Can you work these out from the model? Positions are in its coordinate system, mm. A direction names the side the tool comes from. Coordinates: 2 decimals unless noted, no trailing zeros. Write each loop counter-clockwise with the first axis right and the second up, starting at its lowest first coordinate (ties: lowest second). Pieces come first, ordered by that corner, then holes. Notation, with made-up numbers: M 25.5,31.5 L 83.5,31.5 A22 cw 83.5,56.5 Z; hole C 88,-33 d9. An arc over 180 degrees is marked long. Answer as a JSON object with one key per item and string values. Group by question number.
from build123d import *

# Parameters (mm, degrees)
SKETCH2_W                    = 22.296412808
SKETCH2_H                    = 8
BOSS_EXTRUDE1_DEPTH          = 17.7
CUT_EXTRUDE2_DEPTH           = 5.5
CUT_EXTRUDE3_REACH           = 30.994
SKETCH9_R                    = 1.5
CUT_EXTRUDE4_DEPTH           = 2
M1_2X0_25_TAPPED_HOLE2_D     = 0.95
M1_2X0_25_TAPPED_HOLE2_DEPTH = 2
M1_2X0_25_TAPPED_HOLE2_TIP   = 0.285408794


with BuildPart() as part:
    # Sketch2 → Boss-Extrude1 (new body)
    with BuildSketch(Plane.XY):
        with Locations((11.148206404, 4)):
            Rectangle(SKETCH2_W, SKETCH2_H)
    extrude(amount=BOSS_EXTRUDE1_DEPTH)

    # Sketch3 → Cut-Extrude2 (cut)
    with BuildSketch(Plane.XZ):
        Polygon((0, 15.2), (19.296412808, 15.2), (19.296412808, 10.7), (22.296412808, 10.7), (22.296412808, 7), (19.296412808, 7), (19.296412808, 2.5), (0, 2.5), align=None)
    extrude(amount=-CUT_EXTRUDE2_DEPTH, mode=Mode.SUBTRACT)

    # Sketch4 → Cut-Extrude3 (cut, up to next)
    with BuildSketch(Plane.XZ.offset(-5.5), mode=Mode.PRIVATE) as cut_extrude3_sk1:
        with BuildLine():
            Line((5, 10.070818057), (12.296412808, 10.070818057))
            ThreePointArc((12.296412808, 10.070818057), (13.546412808, 8.820818057), (12.296412808, 7.570818057))
            Line((12.296412808, 7.570818057), (5, 7.570818057))
            ThreePointArc((5, 7.570818057), (3.75, 8.820818057), (5, 10.070818057))
        make_face()
    cut_extrude3_tool1 = extrude(cut_extrude3_sk1.sketch, amount=-CUT_EXTRUDE3_REACH, mode=Mode.PRIVATE) & part.part
    add(cut_extrude3_tool1.solids().sort_by_distance((8.648206, 5.5, 8.820818))[0], mode=Mode.SUBTRACT)

    # Sketch9 → Cut-Extrude4 (cut)
    with BuildSketch(Plane.ZY.offset(-19.296412808)):
        with Locations((4.75, 2.75)):
            Circle(SKETCH9_R)
        with Locations((12.95, 2.75)):
            Circle(SKETCH9_R)
    extrude(amount=-CUT_EXTRUDE4_DEPTH, mode=Mode.SUBTRACT)

    # M1.2x0.25 Tapped Hole2
    with Locations(Plane(origin=(17.296412808, 4, 17.7), x_dir=(1, 0, 0), z_dir=(0, 0, 1))):
        with Locations((0, 0), (-12.293258023, 0)):
            Hole(M1_2X0_25_TAPPED_HOLE2_D / 2, depth=M1_2X0_25_TAPPED_HOLE2_DEPTH)
            with Locations((0, 0, -(M1_2X0_25_TAPPED_HOLE2_DEPTH + M1_2X0_25_TAPPED_HOLE2_TIP / 2))):  # 118° drill point
                Cone(0, M1_2X0_25_TAPPED_HOLE2_D / 2, M1_2X0_25_TAPPED_HOLE2_TIP, mode=Mode.SUBTRACT)


solid = part.part
Q1. If we section it at B-B on z = 4.75: List the corners of the cut face in (x, y) for me.
Q2. If we section it at C-C on x = 15.75: List the corners of the cut face in (y, z) for me.
Q3. If we section it at A-A on y = 2.75: List the corners of the cut face in (x, z) for me.
Q4. Will these pins go through, and if not, where does the flat tip stop? pin 1 (3.5 mm diameter, centred on y = 2, z = 5, fed in from -X); pin 2 (0.9 mm diameter, centred on y = 2.5, z = 4.5, fed in from -X).
Q5. If we section it at D-D on z = 13.5: List the corners of the cut face in (x, y) for me, and give its area (3 significant figures).
Q6. Please list where these lines run through material, in increasing order: L1, parallel to X at y = 4, z = 17.15; L2, parallel to Z at x = 9, y = 3.75; L3, parallel to Z at x = 9.75, y = 7.5.
Q7. We'd pull the mould along X, two halves only. Please class faces 1 (the flat face through (22.296, 6, 9)), 2 (the flat face through (21.296, 3, 13)), 3 (the cylindrical face through (3.75, 6.73, 8.79)), 4 (the flat face through (13, 0, 16)): pulls with the +X half, pulls with the -X half, needs draft (parallel to the pull), parting line crosses it, or undercut.
Q8. On a 3-axis mill with a long thin cutter (end or side, diameter ignored), from which of +Z, -Z, +X, -X, +Y, -Y can I reach the whole of each face in a straight line? I mean faces 5 (the cylindrical face through (20.3, 1.4, 5.4)), 6 (the flat face through (11.3, 5.5, 10.4)), 7 (the flat face through (9, 7, 10.071)). Say none if no direction works.
Reply:
{
 "1": {"outline": "M 0,5.5 L 19.3,5.5 L 19.3,4.25 L 21.3,4.25 L 21.3,1.25 L 19.3,1.25 L 19.3,0 L 22.3,0 L 22.3,8 L 0,8 Z"},
 "2": {"outline": "M 0,0 L 8,0 L 8,17.7 L 0,17.7 L 0,15.2 L 5.5,15.2 L 5.5,2.5 L 0,2.5 Z"},
 "3": {"outline": "M 0,0 L 22.3,0 L 22.3,7 L 19.3,7 L 19.3,6.25 L 21.3,6.25 L 21.3,3.25 L 19.3,3.25 L 19.3,2.5 L 0,2.5 Z; M 0,15.2 L 19.3,15.2 L 19.3,14.45 L 21.3,14.45 L 21.3,11.45 L 19.3,11.45 L 19.3,10.7 L 22.3,10.7 L 22.3,17.7 L 0,17.7 Z"},
 "4": {"pin 1": "x = 19.3", "pin 2": "x = 21.3"},
 "5": {"outline": "M 0,5.5 L 19.3,5.5 L 19.3,4.15 L 21.3,4.15 L 21.3,1.35 L 19.3,1.35 L 19.3,0 L 22.3,0 L 22.3,8 L 0,8 Z", "area": "66.7 mm^2"},
 "6": {"L1": "0 to 4.53, 5.48 to 16.82, 17.77 to 22.3", "L2": "0 to 2.5, 15.2 to 17.7", "L3": "0 to 7.57, 10.07 to 17.7"},
 "7": {"face 1": "pulls with the +X half", "face 2": "pulls with the -X half", "face 3": "undercut", "face 4": "needs draft"},
 "8": {"face 5": "-X", "face 6": "-X, -Y", "face 7": "+Y, -Y"}
}
